Source: three-view drawing plus pictorial views. Frame: mm from the lowest corner of the part. A direction names the side the tool comes from. Coordinates: 2 decimals unless noted, no trailing zeros. Order: outer loops, then holes, each group sorted by start corner. A loop starts at its lowest first (then second) coordinate and runs counter-clockwise, first axis right, second up. Notation, with made-up numbers: (22, 4.25) - (43, 4.25) arc R21 cw to (43, 21.25) - close; hole circle Ø4 at (62, 75.5). An arc over 180 degrees is marked (long way). One line per question, with ' | ' between items.
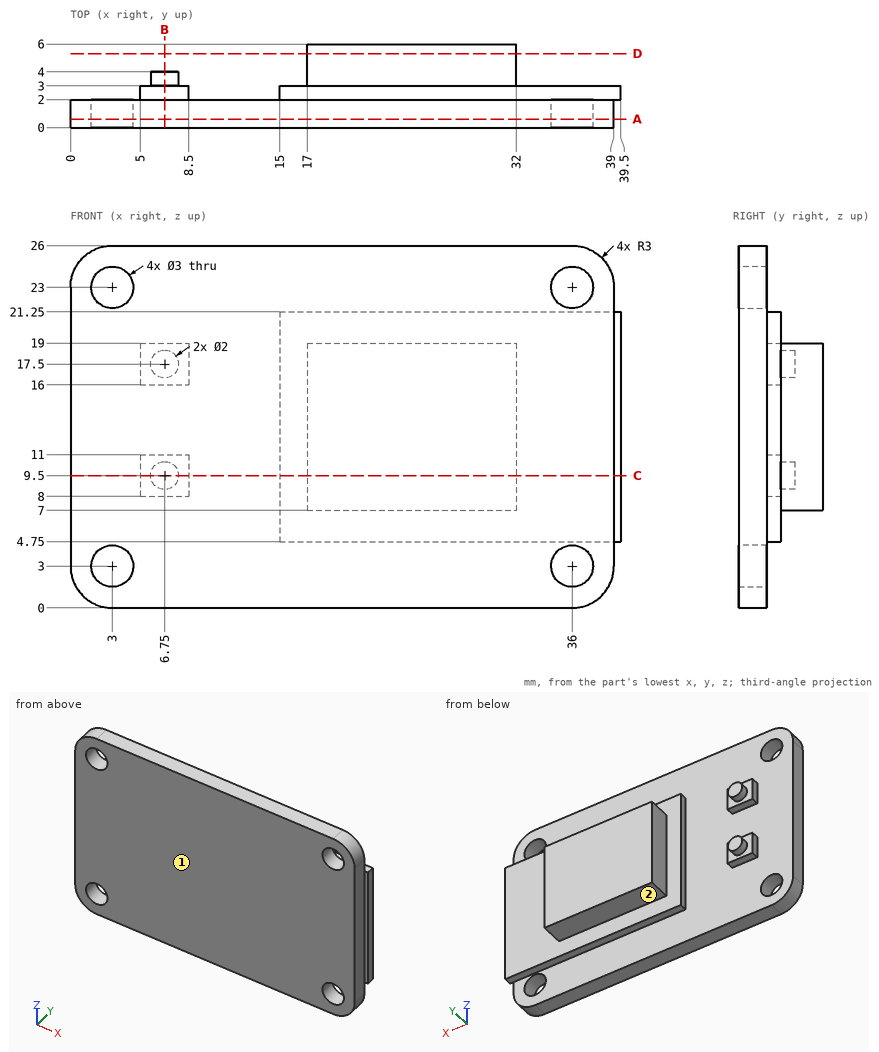
Item 1: Section B-B on x = 6.75. Return the cut outline in (y, z).
Data:
outline: (0, 0) - (2, 0) - (2, 8) - (3, 8) - (3, 8.5) - (4, 8.5) - (4, 10.5) - (3, 10.5) - (3, 11) - (2, 11) - (2, 16) - (3, 16) - (3, 16.5) - (4, 16.5) - (4, 18.5) - (3, 18.5) - (3, 19) - (2, 19) - (2, 26) - (0, 26) - close
Item 2: Access query for the marked faces 1 and 2. Directions: +Z, -Z, +X, -X, +Y, -Y. A direction counts if a zero-diameter tool reaches every point of the face in a straight line with its end or side. Return the directions, or none.
Data:
face 1: +Z, -Z, +X, -X, -Y | face 2: -Z, +X, -X, +Y
Item 3: Section D-D on y = 5.3. Return the cut outline in (x, z), and give its area (3 significant figures).
Data:
outline: (17, 7) - (32, 7) - (32, 19) - (17, 19) - close | area: 180 mm^2
Item 4: Ray query, line 1 (X direction, y = 1.45, z = 3); line 2 (Z direction, x = 7, y = 2.2); line 3 (Y direction, x = 2.5, z = 12.25). Return the intervals inside material, ascending.
Data:
line 1: 0 to 1.5, 4.5 to 34.5, 37.5 to 39 | line 2: 8 to 11, 16 to 19 | line 3: 0 to 2
Item 5: Contact query for flat-ended pins moving along their axis: P1, Ø1, axis at x = 15.5, y = 4, coming from the +Z side (3 decimals); P2, Ø2.5, axis at x = 6.5, z = 17.5, coming from the +Y side; P3, Ø0.8, axis at x = 7.5, y = 2.5, coming from the -Z side; P4, Ø2.5, axis at y = 5, z = 13, coming from the -X side. Output: stop coordinate, or through.
Data:
P1: through | P2: y = 4 | P3: z = 8 | P4: x = 17
Item 6: Section A-A on y = 0.6. Return the cut outline in (x, z), and give its area (3 significant figures).
Data:
outline: (0, 3) arc R3 ccw to (3, 0) - (36, 0) arc R3 ccw to (39, 3) - (39, 23) arc R3 ccw to (36, 26) - (3, 26) arc R3 ccw to (0, 23) - close; hole circle Ø3 at (3, 3); hole circle Ø3 at (3, 23); hole circle Ø3 at (36, 3); hole circle Ø3 at (36, 23) | area: 978 mm^2
Item 7: Section C-C on z = 9.5. Return the cut outline in (x, y).
Data:
outline: (0, 0) - (39, 0) - (39, 2) - (39.5, 2) - (39.5, 3) - (32, 3) - (32, 6) - (17, 6) - (17, 3) - (15, 3) - (15, 2) - (8.5, 2) - (8.5, 3) - (7.75, 3) - (7.75, 4) - (5.75, 4) - (5.75, 3) - (5, 3) - (5, 2) - (0, 2) - close
